Could you check a few things on this model? Use its own coordinates, in mm. Coordinates: 2 decimals unless noted, no trailing zeros. Loops run counter-clockwise (first coordinate to the right, second up) from the corner with the lowest first, then second, coordinate; pieces in that order, holes last.
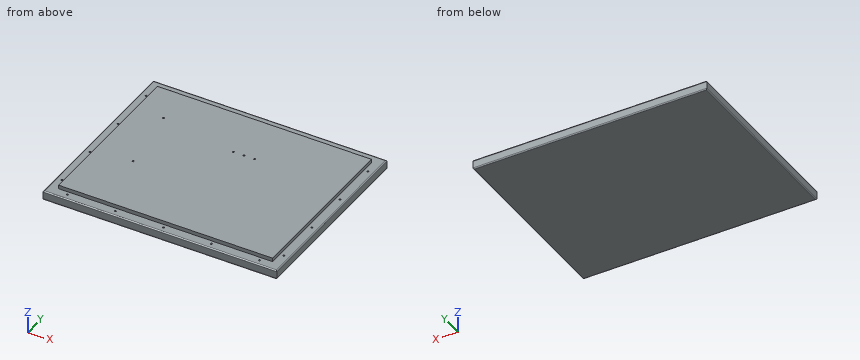
from build123d import *

# Parameters (mm, degrees)
F0_W     = 438
F0_H     = 354
F0_W_2   = 401
F0_H_2   = 317
F1_DEPTH = 17
F2_DEPTH = 24
F3_R     = 2
F4_R     = 2
F6_D     = 3.3
F6_DEPTH = 6.6
F6_TIP   = 0.9914200214
F8_D     = 3.3
F8_DEPTH = 13.5
F8_TIP   = 0.9914200214
F9_D     = 3.3
F9_DEPTH = 13.5
F9_TIP   = 0.9914200214


with BuildPart() as f1:
    # F0 (on Top) → F1 (new body)
    with BuildSketch(Plane.XY):
        with Locations((219, 177)):
            Rectangle(F0_W, F0_H)
        with Locations((219, 177)):
            Rectangle(F0_W_2, F0_H_2, mode=Mode.SUBTRACT)
    extrude(amount=F1_DEPTH)

    # F0 (on Top) → F2 (join)
    with BuildSketch(Plane.XY):
        with Locations((219, 177)):
            Rectangle(F0_W_2, F0_H_2)
    extrude(amount=F2_DEPTH)

    # F3
    f3_edges = [f1.edges().sort_by_distance(p)[0] for p in [
        (0, 177, 0),
        (219, 0, 0),
        (438, 177, 0),
        (219, 354, 0),
    ]]
    fillet(f3_edges, radius=F3_R)

    # F4
    f4_edges = [f1.edges().sort_by_distance(p)[0] for p in [
        (438, 177, 17),
        (219, 0, 17),
        (219, 354, 17),
        (0, 177, 17),
    ]]
    fillet(f4_edges, radius=F4_R)

    # F6
    with Locations(Plane.XY.offset(17)):
        with Locations((11.3, 312), (11.3, 222), (11.3, 132), (11.3, 42), (39, 11.3), (129, 11.3), (219, 11.3), (309, 11.3), (399, 11.3), (426.7, 42), (426.7, 132), (426.7, 222), (426.7, 312), (399, 342.7), (309, 342.7), (219, 342.7), (129, 342.7), (39, 342.7)):
            Hole(F6_D / 2, depth=F6_DEPTH)
            with Locations((0, 0, -(F6_DEPTH + F6_TIP / 2))):  # 118° drill point
                Cone(0, F6_D / 2, F6_TIP, mode=Mode.SUBTRACT)

    # F8
    with Locations(Plane.XY.offset(24)):
        with Locations((216.3, 240.7), (236.3, 240.7), (256.3, 240.7)):
            Hole(F8_D / 2, depth=F8_DEPTH)
            with Locations((0, 0, -(F8_DEPTH + F8_TIP / 2))):  # 118° drill point
                Cone(0, F8_D / 2, F8_TIP, mode=Mode.SUBTRACT)

    # F9
    with Locations(Plane.XY.offset(24)):
        with Locations((71.3, 264.7), (89.3, 136.7)):
            Hole(F9_D / 2, depth=F9_DEPTH)
            with Locations((0, 0, -(F9_DEPTH + F9_TIP / 2))):  # 118° drill point
                Cone(0, F9_D / 2, F9_TIP, mode=Mode.SUBTRACT)


solid = f1.part
1) Imagine slicing it at B-B on y = 180.5. List the corners of the cut face in (x, z) for me, plus the area to 3 significant figures.
2) If I drill on L1, parallel to X at y = 342.7, z = 12.75; L2, parallel to Y at x = 426.7, z = 15.25; L3, parallel to X at y = 222, z = 12.5, over which ranges is the centre line in solid material (lowest first)?
3) Will these pins go through, and if not, where does the flat tip stop? pin 1 (7.5 mm diameter, centred on x = 139.5, z = 19.5, fed in from -Y); pin 2 (2.5 mm diameter, centred on x = 426.7, y = 42, fed in from +Z); pin 3 (10 mm diameter, centred on y = 143, z = 21, fed in from +X).
4) Imagine slicing it at A-A on x = 316. List the corners of the cut face in (y, z) for me, plus the area to 3 significant figures.
Solved:
1. outline: (0, 2) arc R2 ccw to (2, 0) - (436, 0) arc R2 ccw to (438, 2) - (438, 15) arc R2 ccw to (436, 17) - (419.5, 17) - (419.5, 24) - (18.5, 24) - (18.5, 17) - (2, 17) arc R2 ccw to (0, 15) - close
1. area: 10,200 mm2
2. L1: x = 0 to 37.35, 40.65 to 127.35, 130.65 to 217.35, 220.65 to 307.35, 310.65 to 397.35, 400.65 to 438
2. L2: y = 0.02 to 40.35, 43.65 to 130.35, 133.65 to 220.35, 223.65 to 310.35, 313.65 to 353.98
2. L3: x = 0 to 9.65, 12.95 to 425.05, 428.35 to 438
3. pin 1: stops at y = 0.15
3. pin 2: stops at z = 10.16
3. pin 3: stops at x = 437.73
4. outline: (0, 2) arc R2 ccw to (2, 0) - (352, 0) arc R2 ccw to (354, 2) - (354, 15) arc R2 ccw to (352, 17) - (335.5, 17) - (335.5, 24) - (18.5, 24) - (18.5, 17) - (2, 17) arc R2 ccw to (0, 15) - close
4. area: 8,230 mm2
